Part model, mm, in its own coordinate system. A direction names the side the tool comes from. Give positions to 0.01 mm unless a question says otherwise; leave off trailing zeros. Write each loop counter-clockwise with the first axis right and the second up, starting at its lowest first coordinate (ties: lowest second). Pieces come first, ordered by that corner, then holes. Notation, with made-up numbers: M 12.5,74.25 L 34.5,74.25 A7 ccw 34.5,79.25 Z; hole C 52,0 d10. An arc over 180 degrees is marked long. Answer as CSV lines item,"result". Start each with the question number.
1) Mould opens along Z. For faces 1 (the flat face through (-37.96, 0.69, -37.62)), 2 (the cylindrical face through (16.779, 0.708, -10.174)), 3 (the flat face through (-34.73, 0.69, 38.82)) say: pulls with the +Z half, pulls with the -Z half, needs draft (parallel to the pull), parting line crosses it, or undercut.
2) Slice it at D-D, the plane x = -17. Give the cut face in (y, z), plus the area to 3 significant figures.
3) Wall check: line 1 along X through (y, z) = (0.4, 0); line 2 along Z through (x, y) = (1, 0.6); line 3 along Z through (x, y) = (37.5, 0.9). Give the ranges that are in metal, low to high. Write a range as from..to.
4) Slice it at C-C, the plane z = -18. Give the cut face in (x, y).
5) Slice it at A-A, the plane z = 0. Give the cut face in (x, y).
6) Slice it at B-B, the plane x = -3. Give the cut face in (y, z), plus the area to 3 significant figures.
7) Tool access for faces 4 (the cylindrical face through (39.52, 0.69, 31.92)), 5 (the cylindrical face through (26.07, 0.71, 10.02)), 6 (the cylindrical face through (-39.63, 0.69, -31.78)), 7 (the cylindrical face through (-0.348, 0.689, 32.056)): list every direction of +Z, -Z, +X, -X, +Y, -Y with a clear straight run to the whole face (end or side of a thin tool).
8) Pin check, flat tips, straight feed: pin 1 Ø0.7 at (x, y) = (-21.5, 0.5) entering from -Z; pin 2 Ø0.7 at (x, y) = (-1.5, 1) entering from +Z. Stop position of each tip, or through.
```python
from build123d import *

# Parameters (mm, degrees)
SKETCH1_R           = 1.015999997
SKETCH1_R_2         = 1.015999998
BOSS_EXTRUDE1_DEPTH = 1.397
CUT_EXTRUDE1_DEPTH  = 1.397


with BuildPart() as part:
    # Sketch1 → Boss-Extrude1 (new body)
    with BuildSketch(Plane(origin=(0, 0, 0), x_dir=(1, 0, 0), z_dir=(0, 1, 0))):
        with BuildLine():
            Line((39.582900137, 36.114993353), (36.135807663, 39.558338119))
            ThreePointArc((36.135807663, 39.558338119), (35.957741585, 39.627761729), (35.781684056, 39.553391627))
            Line((35.781684056, 39.553391627), (33.985632879, 37.75734045))
            ThreePointArc((33.985632879, 37.75734045), (31.864995739, 39.563392759), (29.648553616, 41.25049416))
            ThreePointArc((29.648553616, 41.25049416), (26.08463695, 42.240855836), (22.7274362, 40.687948442))
            ThreePointArc((22.7274362, 40.687948442), (0, 32.054645119), (-22.7274362, 40.687948442))
            ThreePointArc((-22.7274362, 40.687948442), (-26.08463695, 42.240855836), (-29.648553616, 41.25049416))
            ThreePointArc((-29.648553616, 41.25049416), (-31.979190339, 39.471146237), (-34.203281642, 37.560291864))
            Line((-34.203281642, 37.560291864), (-35.891842785, 39.288069847))
            ThreePointArc((-35.891842785, 39.288069847), (-36.070582137, 39.364521411), (-36.251029365, 39.292193022))
            Line((-36.251029365, 39.292193022), (-39.722106603, 35.899901777))
            ThreePointArc((-39.722106603, 35.899901777), (-39.798570717, 35.719704686), (-39.724180022, 35.538641777))
            Line((-39.724180022, 35.538641777), (-37.952779126, 33.76724088))
            ThreePointArc((-37.952779126, 33.76724088), (-39.65514495, 31.750739818), (-41.25049416, 29.648553616))
            ThreePointArc((-41.25049416, 29.648553616), (-42.240855836, 26.08463695), (-40.687948442, 22.7274362))
            ThreePointArc((-40.687948442, 22.7274362), (-32.054645119, 0), (-40.687948442, -22.7274362))
            ThreePointArc((-40.687948442, -22.7274362), (-42.240855836, -26.08463695), (-41.25049416, -29.648553616))
            ThreePointArc((-41.25049416, -29.648553616), (-39.491481287, -31.954074947), (-37.603777167, -34.155467245))
            Line((-37.603777167, -34.155467245), (-39.342333505, -35.894023583))
            ThreePointArc((-39.342333505, -35.894023583), (-39.416724199, -36.072170919), (-39.34438326, -36.251160408))
            Line((-39.34438326, -36.251160408), (-35.996846779, -39.67644344))
            ThreePointArc((-35.996846779, -39.67644344), (-35.8116648, -39.777312417), (-35.614113895, -39.703552292))
            Line((-35.614113895, -39.703552292), (-33.818062671, -37.907501068))
            ThreePointArc((-33.818062671, -37.907501068), (-31.777299231, -39.633864984), (-29.648553616, -41.25049416))
            ThreePointArc((-29.648553616, -41.25049416), (-26.08463695, -42.240855836), (-22.7274362, -40.687948442))
            ThreePointArc((-22.7274362, -40.687948442), (0, -32.054645119), (22.7274362, -40.687948442))
            ThreePointArc((22.7274362, -40.687948442), (26.08463695, -42.240855836), (29.648553616, -41.25049416))
            ThreePointArc((29.648553616, -41.25049416), (31.839816037, -39.583659694), (33.937557164, -37.800558378))
            Line((33.937557164, -37.800558378), (35.712874192, -39.617107153))
            ThreePointArc((35.712874192, -39.617107153), (35.89865706, -39.693541904), (36.081857691, -39.611109667))
            Line((36.081857691, -39.611109667), (39.53818925, -36.154778109))
            ThreePointArc((39.53818925, -36.154778109), (39.581113192, -35.9880354), (39.507835585, -35.832227866))
            Line((39.507835585, -35.832227866), (37.71178436, -34.036176641))
            ThreePointArc((37.71178436, -34.036176641), (39.542043021, -31.891485286), (41.25049416, -29.648553616))
            ThreePointArc((41.25049416, -29.648553616), (42.240855836, -26.08463695), (40.687948442, -22.7274362))
            ThreePointArc((40.687948442, -22.7274362), (32.054645119, 0), (40.687948442, 22.7274362))
            ThreePointArc((40.687948442, 22.7274362), (42.240855836, 26.08463695), (41.25049416, 29.648553616))
            ThreePointArc((41.25049416, 29.648553616), (39.563392759, 31.864995739), (37.75734045, 33.985632879))
            Line((37.75734045, 33.985632879), (39.573889176, 35.76094986))
            ThreePointArc((39.573889176, 35.76094986), (39.650275245, 35.936142133), (39.582900137, 36.114993353))
        make_face()
        with Locations((-28.220170249, 36.841216125)):
            Circle(SKETCH1_R, mode=Mode.SUBTRACT)
        with Locations((-36.841216125, 28.220170249)):
            Circle(SKETCH1_R, mode=Mode.SUBTRACT)
        with Locations((-24.24546392, 24.24546392)):
            Circle(SKETCH1_R_2, mode=Mode.SUBTRACT)
        with Locations((28.220170249, 36.841216125)):
            Circle(SKETCH1_R, mode=Mode.SUBTRACT)
        with Locations((36.841216125, 28.220170249)):
            Circle(SKETCH1_R, mode=Mode.SUBTRACT)
        with Locations((24.24546392, 24.24546392)):
            Circle(SKETCH1_R_2, mode=Mode.SUBTRACT)
        with Locations((36.841216125, -28.220170249)):
            Circle(SKETCH1_R, mode=Mode.SUBTRACT)
        with Locations((28.220170249, -36.841216125)):
            Circle(SKETCH1_R, mode=Mode.SUBTRACT)
        with Locations((24.24546392, -24.24546392)):
            Circle(SKETCH1_R_2, mode=Mode.SUBTRACT)
        with Locations((-28.220170249, -36.841216125)):
            Circle(SKETCH1_R, mode=Mode.SUBTRACT)
        with Locations((-36.841216125, -28.220170249)):
            Circle(SKETCH1_R, mode=Mode.SUBTRACT)
        with Locations((-24.24546392, -24.24546392)):
            Circle(SKETCH1_R_2, mode=Mode.SUBTRACT)
    extrude(amount=BOSS_EXTRUDE1_DEPTH)

    # Sketch3 → Cut-Extrude1 (cut)
    with BuildSketch(Plane(origin=(0, 1.397, 0), x_dir=(1, 0, 0), z_dir=(0, 1, 0))):
        with BuildLine():
            Line((26.924, 8.076), (26.924, -7.924))
            ThreePointArc((26.924, -7.924), (26.045320344, -10.045320344), (23.924, -10.924))
            Line((23.924, -10.924), (18.924, -10.924))
            ThreePointArc((18.924, -10.924), (16.802679656, -10.045320344), (15.924, -7.924))
            Line((15.924, -7.924), (15.924, 8.076))
            ThreePointArc((15.924, 8.076), (16.802679656, 10.197320344), (18.924, 11.076))
            Line((18.924, 11.076), (23.924, 11.076))
            ThreePointArc((23.924, 11.076), (26.045320344, 10.197320344), (26.924, 8.076))
        make_face()
        with BuildLine():
            Line((-8, 27), (8, 27))
            ThreePointArc((8, 27), (10.121320344, 26.121320344), (11, 24))
            Line((11, 24), (11, 19))
            ThreePointArc((11, 19), (10.121320344, 16.878679656), (8, 16))
            Line((8, 16), (-8, 16))
            ThreePointArc((-8, 16), (-10.121320344, 16.878679656), (-11, 19))
            Line((-11, 19), (-11, 24))
            ThreePointArc((-11, 24), (-10.121320344, 26.121320344), (-8, 27))
        make_face()
        with BuildLine():
            Line((8, -26.848), (-8, -26.848))
            ThreePointArc((-8, -26.848), (-10.121320344, -25.969320344), (-11, -23.848))
            Line((-11, -23.848), (-11, -18.848))
            ThreePointArc((-11, -18.848), (-10.121320344, -16.726679656), (-8, -15.848))
            Line((-8, -15.848), (8, -15.848))
            ThreePointArc((8, -15.848), (10.121320344, -16.726679656), (11, -18.848))
            Line((11, -18.848), (11, -23.848))
            ThreePointArc((11, -23.848), (10.121320344, -25.969320344), (8, -26.848))
        make_face()
        with BuildLine():
            Line((-26.924, -7.924), (-26.924, 8.076))
            ThreePointArc((-26.924, 8.076), (-26.045320344, 10.197320344), (-23.924, 11.076))
            Line((-23.924, 11.076), (-18.924, 11.076))
            ThreePointArc((-18.924, 11.076), (-16.802679656, 10.197320344), (-15.924, 8.076))
            Line((-15.924, 8.076), (-15.924, -7.924))
            ThreePointArc((-15.924, -7.924), (-16.802679656, -10.045320344), (-18.924, -10.924))
            Line((-18.924, -10.924), (-23.924, -10.924))
            ThreePointArc((-23.924, -10.924), (-26.045320344, -10.045320344), (-26.924, -7.924))
        make_face()
    extrude(amount=-CUT_EXTRUDE1_DEPTH, mode=Mode.SUBTRACT)


solid = part.part
```
Found:
1,face 1,"pulls with the -Z half"
1,face 2,"undercut"
1,face 3,"pulls with the +Z half"
2,outline,"M 0,-36.57 L 1.4,-36.57 L 1.4,-10.38 L 0,-10.38 Z; M 0,10.23 L 1.4,10.23 L 1.4,36.57 L 0,36.57 Z"
2,area,"73.4 mm²"
3,line 1,"-32.05..-26.92, -15.92..15.92, 26.92..32.05"
3,line 2,"-32.07..-27, -16..15.85, 26.85..32.07"
3,line 3,"-38.2..-28.99, -27.45..-18.52, 18.52..27.45, 28.99..38.19"
4,outline,"M -37.17,0 L -10.83,0 L -10.83,1.4 L -37.17,1.4 Z; M 10.83,0 L 37.17,0 L 37.17,1.4 L 10.83,1.4 Z"
5,outline,"M -32.05,0 L -26.92,0 L -26.92,1.4 L -32.05,1.4 Z; M -15.92,0 L 15.92,0 L 15.92,1.4 L -15.92,1.4 Z; M 26.92,0 L 32.05,0 L 32.05,1.4 L 26.92,1.4 Z"
6,outline,"M 0,-32.19 L 1.4,-32.19 L 1.4,-27 L 0,-27 Z; M 0,-16 L 1.4,-16 L 1.4,15.85 L 0,15.85 Z; M 0,26.85 L 1.4,26.85 L 1.4,32.19 L 0,32.19 Z"
6,area,"59.2 mm²"
7,face 4,"+X, +Y, -Y"
7,face 5,"+Y, -Y"
7,face 6,"-X, +Y, -Y"
7,face 7,"+Z, +Y, -Y"
8,pin 1,"z = -39.94"
8,pin 2,"z = 32.1"
